Answer from the drawing. Dimensions are ordinates in mm from the lowest x, y and z of the part. A direction names the side the tool comes from. Round coordinates to 2 decimals unless told otherwise and drop trailing zeros. Loops run counter-clockwise (first coordinate to the right, second up) from the corner with the lowest first, then second, coordinate; pieces in that order, holes last.
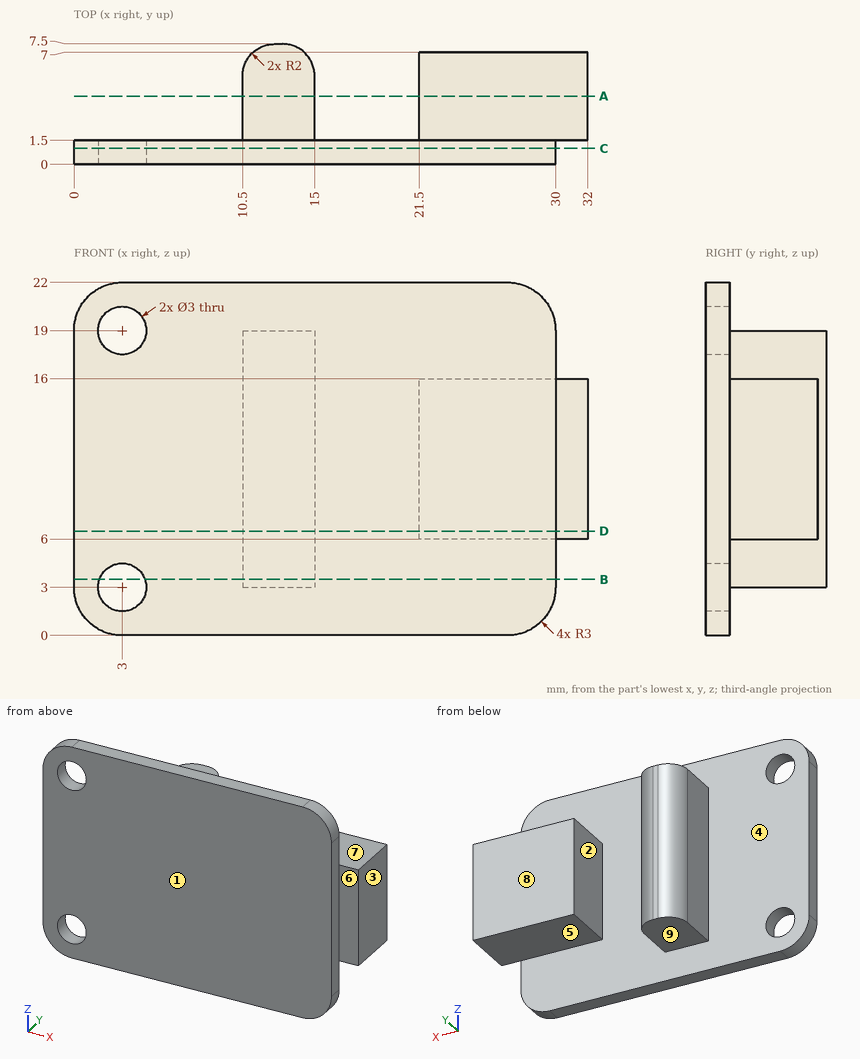
Item 1: Section A-A, the plane y = 4.25 is taken. Give the vertices of the cut face in (x, z).
Item 2: Section D-D, the plane z = 6.5 is taken. Give the vertices of the cut face in (x, y).
Item 3: Determine the mould class of the marked faces 1, 2, 3 and 4 for opening direction X: pulls with the +X half, pulls with the -X half, needs draft (parallel to the pull), parting line crosses it, or undercut.
Item 4: Straight lines are drawn through the part: line 1 (X direction, y = 0.4, z = 19); line 2 (Y direction, x = 28.5, z = 11.5); line 3 (Y direction, x = 16.5, z = 11.5). For each, find the intervals that lie inside material, in ascending order.
Item 5: Each of these flat-tipped pins is pushed along its axis until it touches: P1, Ø8, axis at x = 25, z = 16.5, coming from the -Y side; P2, Ø1.5, axis at x = 11, y = 6.5, coming from the +Z side; P3, Ø1.6, axis at x = 25.5, y = 4.5, coming from the +Z side; P4, Ø5, axis at x = 28.5, z = 13, coming from the +Y side. Where does it stop, or does it pass through?
Item 6: Section B-B, the plane z = 3.5 is taken. Give the vertices of the cut face in (x, y).
Item 7: Section C-C, the plane y = 1 is taken. Give the vertices of the cut face in (x, z).
Item 8: For the marked faces 5, 6, 7, 8 and 9, determine the directions among +Z, -Z, +X, -X, +Y, -Y from which every point of the face is accessible in a straight line to the end or side of a thin tool.
Answer below:
1. outline: (10.5, 3) - (15, 3) - (15, 19) - (10.5, 19) - close; (21.5, 6) - (32, 6) - (32, 16) - (21.5, 16) - close
2. outline: (0, 0) - (30, 0) - (30, 1.5) - (32, 1.5) - (32, 7) - (21.5, 7) - (21.5, 1.5) - (15, 1.5) - (15, 5.5) arc R2 ccw to (13, 7.5) - (12.5, 7.5) arc R2 ccw to (10.5, 5.5) - (10.5, 1.5) - (0, 1.5) - close
3. face 1: needs draft
3. face 2: undercut
3. face 3: pulls with the +X half
3. face 4: undercut
4. line 1: x = 0 to 1.5, 4.5 to 30
4. line 2: y = 0 to 7
4. line 3: y = 0 to 1.5
5. P1: stops at y = 0
5. P2: stops at z = 19
5. P3: stops at z = 16
5. P4: stops at y = 7
6. outline: (0, 0) - (1.59, 0) - (1.59, 1.5) - (0, 1.5) - close; (4.41, 0) - (30, 0) - (30, 1.5) - (15, 1.5) - (15, 5.5) arc R2 ccw to (13, 7.5) - (12.5, 7.5) arc R2 ccw to (10.5, 5.5) - (10.5, 1.5) - (4.41, 1.5) - close
7. outline: (0, 3) arc R3 ccw to (3, 0) - (27, 0) arc R3 ccw to (30, 3) - (30, 19) arc R3 ccw to (27, 22) - (3, 22) arc R3 ccw to (0, 19) - close; hole circle Ø3 at (3, 3); hole circle Ø3 at (3, 19)
8. face 5: -Z, +X, +Y
8. face 6: +Z, -Z, +X, -Y
8. face 7: +Z, +X, +Y
8. face 8: +Z, -Z, +X, +Y
8. face 9: -Z, +X, -X, +Y
